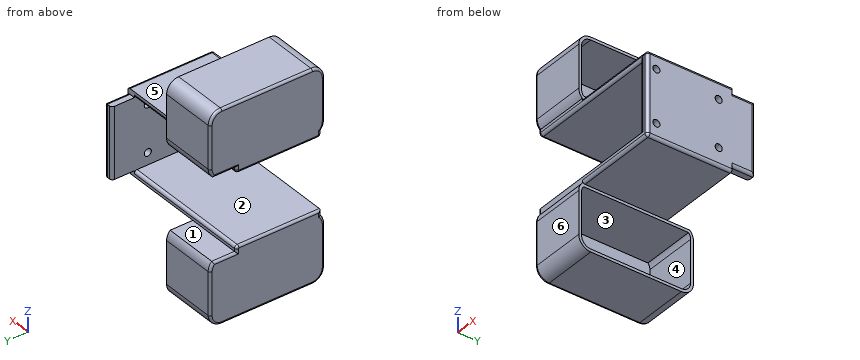
from build123d import *

# Parameters (mm, degrees)
SKETCH_1_W      = 25
SKETCH_1_H      = 38
SKETCH_1_R      = 1.25
EXTRUDE_2_DEPTH = 3
SKETCH_2_W      = 2
SKETCH_2_H      = 30
EXTRUDE_3_DEPTH = 50
EXTRUDE_6_DEPTH = 20
EXTRUDE_7_DEPTH = 1.2
FILLET_4_R      = 1
FILLET_5_R      = 0.8


with BuildPart() as part:
    # 草图1 → 凸台-拉伸2 (new body)
    with BuildSketch(Plane(origin=(0, 0, 0), x_dir=(0, 0, -1), z_dir=(1, 0, 0))):
        Rectangle(SKETCH_1_W, SKETCH_1_H)
        with Locations((9.25, -15.75)):
            Circle(SKETCH_1_R, mode=Mode.SUBTRACT)
        with Locations((8.25, 6.25)):
            Circle(SKETCH_1_R, mode=Mode.SUBTRACT)
        with Locations(Location((-9.25, -15.75, 0), (0, 0, 180))):
            Circle(SKETCH_1_R, mode=Mode.SUBTRACT)
        with Locations(Location((-8.25, 6.25, 0), (0, 0, 180))):
            Circle(SKETCH_1_R, mode=Mode.SUBTRACT)
    extrude(amount=EXTRUDE_2_DEPTH)

    # 草图2 → 凸台-拉伸3 (add)
    with BuildSketch(Plane(origin=(3, 0, 0), x_dir=(0, 0, -1), z_dir=(1, 0, 0))):
        with Locations((13.5, -4)):
            Rectangle(SKETCH_2_W, SKETCH_2_H)
        with Locations((-13.5, -4)):
            Rectangle(SKETCH_2_W, SKETCH_2_H)
    extrude(amount=-EXTRUDE_3_DEPTH)

    # 草图4 → 凸台-拉伸6 (add)
    # profile 1 of 2: a face of its own
    with BuildSketch(Plane.ZY.offset(47)):
        with BuildLine():
            Line((-14.5, 11), (-14.5, 19))
            ThreePointArc((-14.5, 19), (-15.8764117, 19.919688895), (-17.5, 20.242640687))
            Line((-17.5, 20.242640687), (-32.5, 20.242640687))
            ThreePointArc((-32.5, 20.242640687), (-35.5, 19), (-36.742640687, 16))
            Line((-36.742640687, 16), (-36.742640687, -16))
            ThreePointArc((-36.742640687, -16), (-35.5, -19), (-32.5, -20.242640687))
            Line((-32.5, -20.242640687), (-17.5, -20.242640687))
            ThreePointArc((-17.5, -20.242640687), (-15.8764117, -19.919688895), (-14.5, -19))
            Line((-14.5, -19), (-14.5, 11))
        make_face()
        with BuildLine():
            Line((-32.5, 19.242640687), (-25, 19.242640687))
            Line((-25, 19.242640687), (-17.5, 19.242640687))
            ThreePointArc((-17.5, 19.242640687), (-16.442120098, 19.065225724), (-15.5, 18.552394685))
            Line((-15.5, 18.552394685), (-15.5, -12.035462258))
            Line((-15.5, -12.035462258), (-15.5, -18.552394685))
            ThreePointArc((-15.5, -18.552394685), (-16.442120098, -19.065225724), (-17.5, -19.242640687))
            Line((-17.5, -19.242640687), (-31.503062925, -19.242640687))
            Line((-31.503062925, -19.242640687), (-32.5, -19.242640687))
            ThreePointArc((-32.5, -19.242640687), (-34.792893219, -18.292893219), (-35.742640687, -16))
            Line((-35.742640687, -16), (-35.742640687, -12.035462258))
            Line((-35.742640687, -12.035462258), (-35.742640687, 16))
            ThreePointArc((-35.742640687, 16), (-34.792893219, 18.292893219), (-32.5, 19.242640687))
        make_face(mode=Mode.SUBTRACT)
    # profile 2 of 2: a face of its own
    with BuildSketch(Plane.ZY.offset(47)):
        with BuildLine():
            Line((14.5, -19), (14.5, 11))
            Line((14.5, 11), (14.5, 19))
            ThreePointArc((14.5, 19), (15.8764117, 19.919688895), (17.5, 20.242640687))
            Line((17.5, 20.242640687), (32.5, 20.242640687))
            ThreePointArc((32.5, 20.242640687), (35.5, 19), (36.742640687, 16))
            Line((36.742640687, 16), (36.742640687, -16))
            ThreePointArc((36.742640687, -16), (35.5, -19), (32.5, -20.242640687))
            Line((32.5, -20.242640687), (17.5, -20.242640687))
            ThreePointArc((17.5, -20.242640687), (15.8764117, -19.919688895), (14.5, -19))
        make_face()
        with BuildLine():
            Line((35.742640687, -12.035462258), (35.742640687, 16))
            ThreePointArc((35.742640687, 16), (34.792893219, 18.292893219), (32.5, 19.242640687))
            Line((32.5, 19.242640687), (25, 19.242640687))
            Line((25, 19.242640687), (17.5, 19.242640687))
            ThreePointArc((17.5, 19.242640687), (16.442120098, 19.065225724), (15.5, 18.552394685))
            Line((15.5, 18.552394685), (15.5, -12.035462258))
            Line((15.5, -12.035462258), (15.5, -18.552394685))
            ThreePointArc((15.5, -18.552394685), (16.442120098, -19.065225724), (17.5, -19.242640687))
            Line((17.5, -19.242640687), (31.503062925, -19.242640687))
            Line((31.503062925, -19.242640687), (32.5, -19.242640687))
            ThreePointArc((32.5, -19.242640687), (34.792893219, -18.292893219), (35.742640687, -16))
            Line((35.742640687, -16), (35.742640687, -12.035462258))
        make_face(mode=Mode.SUBTRACT)
    extrude(amount=-EXTRUDE_6_DEPTH)

    # 草图5 → 凸台-拉伸7 (add)
    with BuildSketch(Plane.ZY.offset(47)):
        with BuildLine():
            Line((-32.5, 19.242640687), (-17.5, 19.242640687))
            ThreePointArc((-17.5, 19.242640687), (-16.442120098, 19.065225724), (-15.5, 18.552394685))
            Line((-15.5, 18.552394685), (-15.5, -18.552394685))
            ThreePointArc((-15.5, -18.552394685), (-16.442120098, -19.065225724), (-17.5, -19.242640687))
            Line((-17.5, -19.242640687), (-32.5, -19.242640687))
            ThreePointArc((-32.5, -19.242640687), (-34.792893219, -18.292893219), (-35.742640687, -16))
            Line((-35.742640687, -16), (-35.742640687, 16))
            ThreePointArc((-35.742640687, 16), (-34.792893219, 18.292893219), (-32.5, 19.242640687))
        make_face()
        with BuildLine():
            Line((35.742640687, -16), (35.742640687, 16))
            ThreePointArc((35.742640687, 16), (34.792893219, 18.292893219), (32.5, 19.242640687))
            Line((32.5, 19.242640687), (17.5, 19.242640687))
            ThreePointArc((17.5, 19.242640687), (16.442120098, 19.065225724), (15.5, 18.552394685))
            Line((15.5, 18.552394685), (15.5, -18.552394685))
            ThreePointArc((15.5, -18.552394685), (16.442120098, -19.065225724), (17.5, -19.242640687))
            Line((17.5, -19.242640687), (32.5, -19.242640687))
            ThreePointArc((32.5, -19.242640687), (34.792893219, -18.292893219), (35.742640687, -16))
        make_face()
    extrude(amount=-EXTRUDE_7_DEPTH)

    # 圆角4
    fillet_4_edges = [part.edges().sort_by_distance(p)[0] for p in [
        (-23.5, -19, 12.5),
        (-12, -19, 14.5),
        (-12, -19, -14.5),
        (0, -19, 0),
        (0, 19, 0),
        (-23.5, 11, -12.5),
        (-23.5, 11, 12.5),
        (3, -19, 0),
        (3, 15, 12.5),
        (3, -4, 14.5),
        (3, -4, -14.5),
        (3, 15, -12.5),
        (3, 19, 0),
    ]]
    fillet(fillet_4_edges, radius=FILLET_4_R - 0.0001)  # a hair under: the kernel refuses the full size

    # 圆角5
    fillet_5_edges = [part.edges().sort_by_distance(p)[0] for p in [
        (-47, -19.919688895, 15.8764117),
        (-47, -20.242640687, 25),
        (-47, -19, 35.5),
        (-47, 0, 36.742640687),
        (-47, 19, 35.5),
        (-47, 20.242640687, 25),
        (-47, 19.919688895, 15.8764117),
        (-47, 15, 14.5),
        (-47, -4, 12.5),
        (-47, 11, 13.99995),
        (-47, 10.707136071, 12.792863929),
        (-47, -18.707136071, 12.792863929),
        (-47, -4.49995, -12.5),
        (-47, 10.707136071, -12.792863929),
        (-47, 11, -13.99995),
        (-47, -19, -13.5),
        (-47, -19, 13.99995),
        (-47, 19.919688895, -15.8764117),
        (-47, 20.242640687, -25),
        (-47, 19, -35.5),
        (-47, 0, -36.742640687),
        (-47, -19, -35.5),
        (-47, -20.242640687, -25),
        (-47, -19.919688895, -15.8764117),
        (-47, 15, -14.5),
    ]]
    fillet(fillet_5_edges, radius=FILLET_5_R)


solid = part.part
Could you check a few things on this model? Use its own coordinates, in mm. Face numbers are marked on the shaded views. A direction names the side the tool comes from. Give positions to 0.01 mm unless a question says otherwise; leave off trailing zeros. Order: outer loops, then holes, each group sorted by start corner. A loop starts at its lowest first (then second) coordinate and runs counter-clockwise, first axis right, second up.
1. For the marked faces 1, 2 and 3, which set-ups out of +Z, -Z, +X, -X, +Y, -Y let a thin tool reach every point of the face, with its end or its side?
2. Will these pins go through, and if not, where does the flat tip stop? P1, Ø4, axis at y = 1.5, z = 20, coming from the +X side; P2, Ø5, axis at y = 3, z = -16.5, coming from the +X side; P3, Ø2, axis at y = 6.25, z = -8.25, coming from the +X side; P4, Ø2, axis at x = 1, y = 15.5, coming from the -Z side.
3. Suppose I cut it at D-D (y = 4). List the corners of the cut face in (x, z) for me.
4. Suppose I cut it at C-C (x = -32.5). Give the number of separate pieces and of enclosed holes in the cut face, plus the area to 3 significant figures.
5. I need wall thicknesses on L1, parallel to Z at x = -30.5, y = -8; L2, parallel to Y at x = -37, z = 20; L3, parallel to Y at x = 1.3, z = 9.25. Which ranges of each line are inside material? Lowest first, please.
6. Suppose I cut it at A-A (y = 12.5). List the corners of the cut face in (x, z) for me, plus the area to 3 significant figures.
7. We'd pull the mould along Y, two halves only. Please class the marked faces 4, 5 and 6: pulls with the +Y half, pulls with the -Y half, needs draft (parallel to the pull), parting line crosses it, or undercut.
Solved:
1. face 1: +X, -X, +Y
1. face 2: -X, +Y, -Y
1. face 3: +X
2. P1: stops at x = -45.8
2. P2: stops at x = 2.87
2. P3: passes through
2. P4: stops at z = -12.5
3. outline: (-47, -35.94) arc R0.8 ccw to (-46.2, -36.74) - (-27, -36.74) - (-27, -35.74) - (-45.8, -35.74) - (-45.8, -15.5) - (-27, -15.5) - (-27, -14.5) - (2, -14.5) arc R1 ccw to (3, -13.5) - (3, 13.5) arc R1 ccw to (2, 14.5) - (-27, 14.5) - (-27, 15.5) - (-45.8, 15.5) - (-45.8, 35.74) - (-27, 35.74) - (-27, 36.74) - (-46.2, 36.74) arc R0.8 ccw to (-47, 35.94) - (-47, 13.3) arc R0.8 ccw to (-46.2, 12.5) - (0, 12.5) - (0, -12.5) - (-46.2, -12.5) arc R0.8 ccw to (-47, -13.3) - close
4. separate pieces: 2
4. enclosed holes: 2
4. area: 353 mm2
5. L1: z = -36.74 to -35.74, -15.5 to -12.5, 12.5 to 15.5, 35.74 to 36.74
5. L2: y = -20.24 to -19.24, 19.24 to 20.24
5. L3: y = -19 to -17, -14.5 to 5.5, 7 to 19
6. outline: (-47, -35.94) arc R0.8 ccw to (-46.2, -36.74) - (-27, -36.74) - (-27, -35.74) - (-45.8, -35.74) - (-45.8, -15.5) - (-27, -15.5) - (-27, -14.5) - (-46.2, -14.5) arc R0.8 ccw to (-47, -15.3) - close; (-47, 15.3) arc R0.8 ccw to (-46.2, 14.5) - (-27, 14.5) - (-27, 15.5) - (-45.8, 15.5) - (-45.8, 35.74) - (-27, 35.74) - (-27, 36.74) - (-46.2, 36.74) arc R0.8 ccw to (-47, 35.94) - close; (0, -12.5) - (2, -12.5) arc R1 ccw to (3, -11.5) - (3, 11.5) arc R1 ccw to (2, 12.5) - (0, 12.5) - close
6. area: 203 mm2
7. face 4: undercut
7. face 5: needs draft
7. face 6: pulls with the -Y half
